from build123d import *

# Parameters (mm, degrees)
EXTRUDE_1_DEPTH     = 20
EXTRUDE_2_DEPTH     = 4
SKETCH_3_R          = 2.6
CUT_EXTRUDE_1_DEPTH = 54.38539126
SKETCH_4_R          = 2.6
CUT_EXTRUDE_2_DEPTH = 54.38539126
EXTRUDE_START       = -10
EXTRUDE_3_DEPTH     = 2.9
FILLET_1_R          = 0.5
CHAMFER_1_SIZE      = 1


with BuildPart() as part:
    # Эскиз1 → Бобышка-Вытянуть1 (new, symmetric)
    with BuildSketch(Plane.XY):
        Polygon((0, 0), (0, -35), (-4, -35), (-4, 4), (35, 4), (35, 0), align=None)
    extrude(amount=EXTRUDE_1_DEPTH, both=True)

    # Эскиз2 → Бобышка-Вытянуть2 (add)
    with BuildSketch(Plane.XY.offset(20)):
        Polygon((0, -35), (0, 0), (35, 0), align=None)
    extrude_2 = extrude(amount=-EXTRUDE_2_DEPTH)

    # Зеркальное отражение1: Бобышка-Вытянуть2 across plane
    add(extrude_2.mirror(Plane.XY))

    # Эскиз3 → Вырез-Вытянуть1 (cut, through all)
    with BuildSketch(Plane(origin=(0, 0, 0), x_dir=(0, 0, -1), z_dir=(1, 0, 0))):
        with Locations((-10, -27.5)):
            Circle(SKETCH_3_R)
        with Locations((10, -27.5)):
            Circle(SKETCH_3_R)
        with Locations((10, -7.5)):
            Circle(SKETCH_3_R)
        with Locations((-10, -7.5)):
            Circle(SKETCH_3_R)
    extrude(amount=-CUT_EXTRUDE_1_DEPTH, mode=Mode.SUBTRACT)

    # Эскиз4 → Вырез-Вытянуть2 (cut, through all)
    with BuildSketch(Plane.XZ):
        with Locations((27.5, -10)):
            Circle(SKETCH_4_R)
        with Locations((7.5, -10)):
            Circle(SKETCH_4_R)
        with Locations((7.5, 10)):
            Circle(SKETCH_4_R)
        with Locations((27.5, 10)):
            Circle(SKETCH_4_R)
    extrude(amount=-CUT_EXTRUDE_2_DEPTH, mode=Mode.SUBTRACT)

    # Эскиз5 → Бобышка-Вытянуть3 (add, symmetric)
    with BuildSketch(Plane.XY.offset(20).offset(EXTRUDE_START)):
        Polygon((-0.888730163, 4), (-3.292893219, 6.404163056), (-6.404163056, 3.292893219), (-4, 0.888730163), (-4, 4), align=None)
        Polygon((35, 3.111269837), (31.707106781, 6.404163056), (30.151471863, 4.848528137), (35, 0), align=None)
        Polygon((-4.848528137, -30.151471863), (0, -35), (-3.111269837, -35), (-6.404163056, -31.707106781), align=None)
    extrude_3 = extrude(amount=EXTRUDE_3_DEPTH, both=True)

    # Зеркальное отражение2: Бобышка-Вытянуть3 across plane
    add(extrude_3.mirror(Plane.XY))

    # Скругление1
    fillet_1_edges = [part.edges().sort_by_distance(p)[0] for p in [
        (-4, -35, 0),
        (-4, 4, 16.45),
        (35, 4, 0),
        (-4, 4, -16.45),
        (-4, 4, 0),
    ]]
    fillet(fillet_1_edges, radius=FILLET_1_R)

    # Фаска1
    chamfer_1_edges = [part.edges().sort_by_distance(p)[0] for p in [
        (0, 0, 0),
        (0, -17.5, 16),
        (17.5, 0, 16),
        (17.5, 0, -16),
        (0, -17.5, -16),
    ]]
    chamfer(chamfer_1_edges, length=CHAMFER_1_SIZE)


solid = part.part
Could you check a few things on this model? Use its own coordinates, in mm. A direction names the side the tool comes from. Round coordinates to 2 decimals unless told otherwise and drop trailing zeros. Order: outer loops, then holes, each group sorted by start corner. A loop starts at its lowest first (then second) coordinate and runs counter-clockwise, first axis right, second up.
(1) Please list where these lines run through material, in increasing order: line 1 along Y through (x, z) = (-1.75, -10); line 2 along Z through (x, y) = (22, -7.5); line 3 along Z through (x, y) = (27.5, 2.55).
Response values:
line 1: y = -35 to -30.1, -24.9 to -10.1, -4.9 to 4.86
line 2: z = -20 to -16, 16 to 20
line 3: z = -20 to -12.6, -7.4 to 7.4, 12.6 to 20
(2) If we mould it in two halves opening along X, with no side actions, what happens to faces 5 (the flat face through (-2.074, 5.185, -9.959)), 6 (the flat face through (-5.22, 2.11, -9.96)), 7 (the flat face through (32, 5, -12.9))? For each: released by +X, released by -X, zero draft, split by the parting line, or undercut.
Response values:
face 5: undercut
face 6: released by -X
face 7: zero draft
(3) Which directions (+Z, -Z, +X, -X, +Y, -Y) give clear straight access to the entire face, cutting with the end or side of a thin tool? Please do faces 1 (the flat face through (30.94, 5.637, -9.959)), 2 (the flat face through (32, 5, 7.1)), 3 (the flat face through (-5.637, -30.94, 10.041)), 4 (the flat face through (18, 0, 0)).
Response values:
face 1: +Z, -Z, +Y
face 2: +X, -X, +Y
face 3: +Z, -Z, -X
face 4: +X, -Y
(4) I'm going to push flat-ended pins straight in: pin 1 (1.2 mm diameter, centred on x = -5.5, y = -32.5, fed in from -Z); pin 2 (1 mm diameter, centred on y = -9, z = 0, fed in from +X); pin 3 (8 mm diameter, centred on y = -29, z = 0, fed in from -X). Where does each tip first touch, or does it pass through?
Response values:
pin 1: stops at z = -12.9
pin 2: stops at x = 0
pin 3: stops at x = -4
(5) Imagine slicing it at D-D (x = 12). Write out the boundary of the cut face in (y, z), plus the area to 3 significant figures.
Response values:
outline: (-23, -20) - (4, -20) - (4, 20) - (-23, 20) - (-23, 16) - (-1, 16) - (0, 15) - (0, -15) - (-1, -16) - (-23, -16) - close
area: 345 mm2
(6) Imagine slicing it at A-A (y = -27.5). Write out the boundary of the cut face in (x, z).
Response values:
outline: (-4, -20) - (7.5, -20) - (7.5, -16) - (1, -16) - (0, -15) - (0, -12.6) - (-4, -12.6) - close; (-4, -7.4) - (0, -7.4) - (0, 7.4) - (-4, 7.4) - close; (-4, 12.6) - (0, 12.6) - (0, 15) - (1, 16) - (7.5, 16) - (7.5, 20) - (-4, 20) - close
(7) Imagine slicing it at B-B (z = -1). Write out the boundary of the cut face in (x, y).
Response values:
outline: (-4, -34.5) arc R0.5 ccw to (-3.5, -35) - (0, -35) - (0, -1) - (1, 0) - (35, 0) - (35, 3.5) arc R0.5 ccw to (34.5, 4) - (-3.5, 4) arc R0.5 ccw to (-4, 3.5) - close
(8) Imagine slicing it at C-C (x = 27.5). Write out the boundary of the cut face in (y, z), plus the area to 3 significant figures.
Response values:
outline: (-7.5, -20) - (4, -20) - (4, -12.6) - (0, -12.6) - (0, -15) - (-1, -16) - (-7.5, -16) - close; (-7.5, 16) - (-1, 16) - (0, 15) - (0, 12.6) - (4, 12.6) - (4, 20) - (-7.5, 20) - close; (0, -7.4) - (4, -7.4) - (4, 7.4) - (0, 7.4) - close
area: 179 mm2
